Check sheet for the drawn part. Datum: minimum x, y, z corner. Units: mm. A direction names the side the tool comes from. Coordinates: 2 decimals unless noted, no trailing zeros. Loops run counter-clockwise (first coordinate to the right, second up) from the corner with the lowest first, then second, coordinate; pieces in that order, holes last. Notation, with made-up numbers: M 17,47 L 25,47 A14 ccw 25,53 Z; hole C 13,-0.75 d3. An arc over 180 degrees is marked long. Answer as CSV lines item,"result". Start each with the question number.
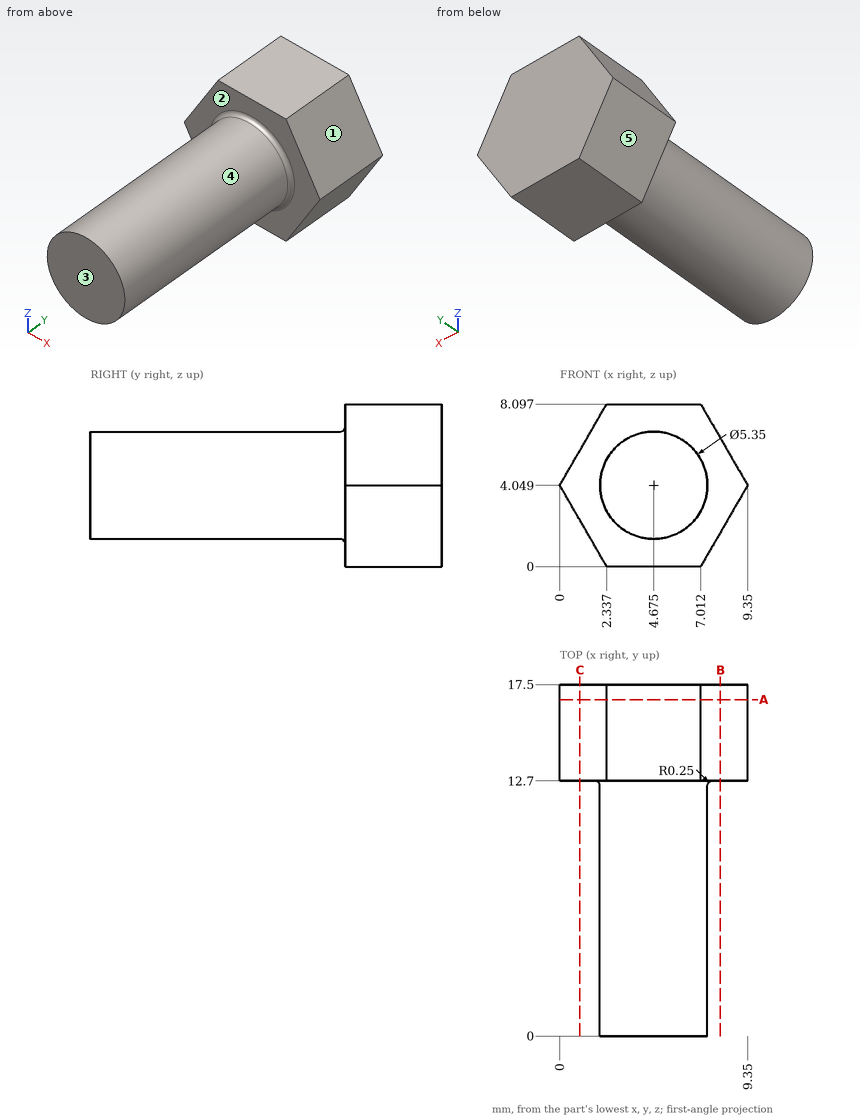
Item 1: Set-up check for the marked faces 1 and 2: record each of +Z, -Z, +X, -X, +Y, -Y from which the full face is reachable in a straight line by a thin tool's end or side.
Item 2: Sectioned sample at C-C, the plane x = 1. Record the boundary of the cut face in (y, z), and give its area (3 significant figures).
Item 3: Sectioned sample at B-B, the plane x = 8. Record the boundary of the cut face in (y, z).
Item 4: Go/stop test with flat-tipped pins: pin 1 (4 mm diameter, centred on y = 8, z = 1, fed in from -X) (1 decimal); pin 2 (1.5 mm diameter, centred on y = 9, z = 5, fed in from +X); pin 3 (2 mm diameter, centred on x = 4.5, y = 4.5, fed in from +Z). Record where each tip stops, or that it passes through.
Item 5: Release check for a two-part mould opening along X. For the marked faces 3, 4 and 5 record: released by +X, released by -X, zero draft, split by the parting line, or undercut.
Item 6: Material ranges on line 1 (Y direction, x = 2, z = 5.25); line 2 (Z direction, x = 4.75, y = 0.5) (1 decimal); line 3 (Z direction, x = 7.25, y = 16) (1 decimal), recorded low to high. Write a range as from..to.
Item 7: Sectioned sample at A-A, the plane y = 16.75. Record the boundary of the cut face in (x, z).
Reply:
1,face 1,"+Z, +X, +Y, -Y"
1,face 2,"-Y"
2,outline,"M 12.7,2.32 L 17.5,2.32 L 17.5,5.78 L 12.7,5.78 Z"
2,area,"16.6 mm²"
3,outline,"M 12.7,1.71 L 17.5,1.71 L 17.5,6.39 L 12.7,6.39 Z"
4,pin 1,"x = 2.2"
4,pin 2,"x = 7.34"
4,pin 3,"z = 6.72"
5,face 3,"zero draft"
5,face 4,"split by the parting line"
5,face 5,"released by -X"
6,line 1,"12.7..17.5"
6,line 2,"1.4..6.7"
6,line 3,"0.4..7.7"
7,outline,"M 0,4.05 L 2.34,0 L 7.01,0 L 9.35,4.05 L 7.01,8.1 L 2.34,8.1 Z"
